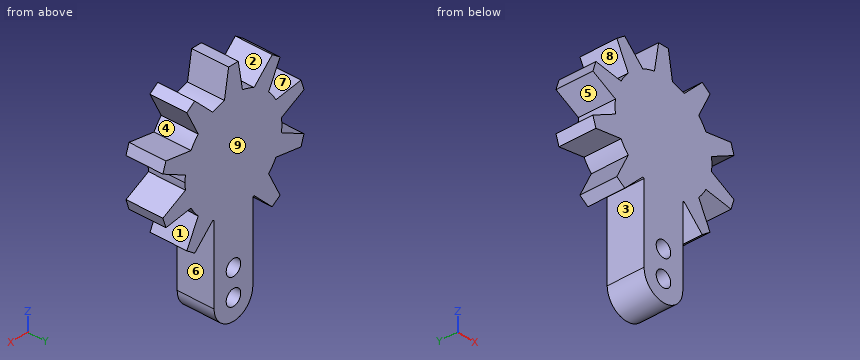
```python
from build123d import *

# Parameters (mm, degrees)
BOSS_EXTRUDE2_DEPTH = 7
SKETCH2_R           = 1.5
BOSS_EXTRUDE3_DEPTH = 7


with BuildPart() as part:
    # Sketch1 → Boss-Extrude2 (new body)
    with BuildSketch(Plane(origin=(0, 0, 0), x_dir=(1, 0, 0), z_dir=(0, 1, 0))):
        with BuildLine():
            Line((-2, 9), (-1.862495894, 9.825024633))
            ThreePointArc((-1.862495894, 9.825024633), (-3.090169944, 9.510565163), (-4.268213752, 9.043359518))
            Line((-4.268213752, 9.043359518), (-3.672033282, 8.456723454))
            Line((-3.672033282, 8.456723454), (-6.908101259, 6.105582445))
            Line((-6.908101259, 6.105582445), (-7.281795413, 6.853864279))
            ThreePointArc((-7.281795413, 6.853864279), (-8.090169944, 5.877852523), (-8.768610817, 4.807438439))
            Line((-8.768610817, 4.807438439), (-7.941474658, 4.683265982))
            Line((-7.941474658, 4.683265982), (-9.177542635, 0.879039917))
            Line((-9.177542635, 0.879039917), (-9.919696584, 1.264760725))
            ThreePointArc((-9.919696584, 1.264760725), (-10, 0), (-9.919696584, -1.264760725))
            Line((-9.919696584, -1.264760725), (-9.177542635, -0.879039917))
            Line((-9.177542635, -0.879039917), (-7.941474658, -4.683265982))
            Line((-7.941474658, -4.683265982), (-8.768610817, -4.807438439))
            ThreePointArc((-8.768610817, -4.807438439), (-8.090169944, -5.877852523), (-7.281795413, -6.853864279))
            Line((-7.281795413, -6.853864279), (-6.908101259, -6.105582445))
            Line((-6.908101259, -6.105582445), (-3.672033282, -8.456723454))
            Line((-3.672033282, -8.456723454), (-4.268213752, -9.043359518))
            ThreePointArc((-4.268213752, -9.043359518), (-3.090169944, -9.510565163), (-1.862495894, -9.825024633))
            Line((-1.862495894, -9.825024633), (-2, -9))
            Line((-2, -9), (2, -9))
            Line((2, -9), (1.862495894, -9.825024633))
            ThreePointArc((1.862495894, -9.825024633), (3.090169944, -9.510565163), (4.268213752, -9.043359518))
            Line((4.268213752, -9.043359518), (3.672033282, -8.456723454))
            Line((3.672033282, -8.456723454), (6.908101259, -6.105582445))
            Line((6.908101259, -6.105582445), (7.281795413, -6.853864279))
            ThreePointArc((7.281795413, -6.853864279), (8.090169944, -5.877852523), (8.768610817, -4.807438439))
            Line((8.768610817, -4.807438439), (7.941474658, -4.683265982))
            Line((7.941474658, -4.683265982), (9.177542635, -0.879039917))
            Line((9.177542635, -0.879039917), (9.919696584, -1.264760725))
            ThreePointArc((9.919696584, -1.264760725), (9.979903953, -0.633653756), (10, 0))
            ThreePointArc((10, 0), (9.979903953, 0.633653756), (9.919696584, 1.264760725))
            Line((9.919696584, 1.264760725), (9.177542635, 0.879039917))
            Line((9.177542635, 0.879039917), (7.941474658, 4.683265982))
            Line((7.941474658, 4.683265982), (8.768610817, 4.807438439))
            ThreePointArc((8.768610817, 4.807438439), (8.090169944, 5.877852523), (7.281795413, 6.853864279))
            Line((7.281795413, 6.853864279), (6.908101259, 6.105582445))
            Line((6.908101259, 6.105582445), (3.672033282, 8.456723454))
            Line((3.672033282, 8.456723454), (4.268213752, 9.043359518))
            ThreePointArc((4.268213752, 9.043359518), (3.090169944, 9.510565163), (1.862495894, 9.825024633))
            Line((1.862495894, 9.825024633), (2, 9))
            Line((2, 9), (-2, 9))
        make_face()
        with BuildLine():
            ThreePointArc((-8.768610817, -4.807438439), (-9.510565163, -3.090169944), (-9.919696584, -1.264760725))
            Line((-9.919696584, -1.264760725), (-14.574864739, -3.684198399))
            Line((-14.574864739, -3.684198399), (-13.95683075, -5.586311432))
            Line((-13.95683075, -5.586311432), (-8.768610817, -4.807438439))
        make_face()
        with BuildLine():
            ThreePointArc((-4.268213752, -9.043359518), (-5.877852523, -8.090169944), (-7.281795413, -6.853864279))
            Line((-7.281795413, -6.853864279), (-9.625795779, -11.547469663))
            Line((-9.625795779, -11.547469663), (-8.00776179, -12.723040168))
            Line((-8.00776179, -12.723040168), (-4.268213752, -9.043359518))
        make_face()
        with BuildLine():
            ThreePointArc((1.862495894, -9.825024633), (0, -10), (-1.862495894, -9.825024633))
            Line((-1.862495894, -9.825024633), (-1, -15))
            Line((-1, -15), (1, -15))
            Line((1, -15), (1.862495894, -9.825024633))
        make_face()
        with BuildLine():
            Line((9.625795779, -11.547469663), (7.281795413, -6.853864279))
            ThreePointArc((7.281795413, -6.853864279), (5.877852523, -8.090169944), (4.268213752, -9.043359518))
            Line((4.268213752, -9.043359518), (8.00776179, -12.723040168))
            Line((8.00776179, -12.723040168), (9.625795779, -11.547469663))
        make_face()
        with BuildLine():
            Line((14.574864739, -3.684198399), (9.919696584, -1.264760725))
            ThreePointArc((9.919696584, -1.264760725), (9.510565163, -3.090169944), (8.768610817, -4.807438439))
            Line((8.768610817, -4.807438439), (13.95683075, -5.586311432))
            Line((13.95683075, -5.586311432), (14.574864739, -3.684198399))
        make_face()
        with BuildLine():
            Line((13.95683075, 5.586311432), (8.768610817, 4.807438439))
            ThreePointArc((8.768610817, 4.807438439), (9.510565163, 3.090169944), (9.919696584, 1.264760725))
            Line((9.919696584, 1.264760725), (14.574864739, 3.684198399))
            Line((14.574864739, 3.684198399), (13.95683075, 5.586311432))
        make_face()
        with BuildLine():
            Line((8.00776179, 12.723040168), (4.268213752, 9.043359518))
            ThreePointArc((4.268213752, 9.043359518), (5.877852523, 8.090169944), (7.281795413, 6.853864279))
            Line((7.281795413, 6.853864279), (9.625795779, 11.547469663))
            Line((9.625795779, 11.547469663), (8.00776179, 12.723040168))
        make_face()
        with BuildLine():
            Line((1, 15), (-1, 15))
            Line((-1, 15), (-1.862495894, 9.825024633))
            ThreePointArc((-1.862495894, 9.825024633), (0, 10), (1.862495894, 9.825024633))
            Line((1.862495894, 9.825024633), (1, 15))
        make_face()
        with BuildLine():
            ThreePointArc((-7.281795413, 6.853864279), (-5.877852523, 8.090169944), (-4.268213752, 9.043359518))
            Line((-4.268213752, 9.043359518), (-8.00776179, 12.723040168))
            Line((-8.00776179, 12.723040168), (-9.625795779, 11.547469663))
            Line((-9.625795779, 11.547469663), (-7.281795413, 6.853864279))
        make_face()
        with BuildLine():
            ThreePointArc((-9.919696584, 1.264760725), (-9.510565163, 3.090169944), (-8.768610817, 4.807438439))
            Line((-8.768610817, 4.807438439), (-13.95683075, 5.586311432))
            Line((-13.95683075, 5.586311432), (-14.574864739, 3.684198399))
            Line((-14.574864739, 3.684198399), (-9.919696584, 1.264760725))
        make_face()
        with BuildLine():
            Line((-7.941474658, 4.683265982), (-8.768610817, 4.807438439))
            ThreePointArc((-8.768610817, 4.807438439), (-9.510565163, 3.090169944), (-9.919696584, 1.264760725))
            Line((-9.919696584, 1.264760725), (-9.177542635, 0.879039917))
            Line((-9.177542635, 0.879039917), (-7.941474658, 4.683265982))
        make_face()
        with BuildLine():
            Line((-2, -9), (-1.862495894, -9.825024633))
            ThreePointArc((-1.862495894, -9.825024633), (0, -10), (1.862495894, -9.825024633))
            Line((1.862495894, -9.825024633), (2, -9))
            Line((2, -9), (-2, -9))
        make_face()
        with BuildLine():
            ThreePointArc((4.268213752, -9.043359518), (5.877852523, -8.090169944), (7.281795413, -6.853864279))
            Line((7.281795413, -6.853864279), (6.908101259, -6.105582445))
            Line((6.908101259, -6.105582445), (3.672033282, -8.456723454))
            Line((3.672033282, -8.456723454), (4.268213752, -9.043359518))
        make_face()
        with BuildLine():
            Line((-6.908101259, -6.105582445), (-7.281795413, -6.853864279))
            ThreePointArc((-7.281795413, -6.853864279), (-5.877852523, -8.090169944), (-4.268213752, -9.043359518))
            Line((-4.268213752, -9.043359518), (-3.672033282, -8.456723454))
            Line((-3.672033282, -8.456723454), (-6.908101259, -6.105582445))
        make_face()
        with BuildLine():
            Line((-9.177542635, -0.879039917), (-9.919696584, -1.264760725))
            ThreePointArc((-9.919696584, -1.264760725), (-9.510565163, -3.090169944), (-8.768610817, -4.807438439))
            Line((-8.768610817, -4.807438439), (-7.941474658, -4.683265982))
            Line((-7.941474658, -4.683265982), (-9.177542635, -0.879039917))
        make_face()
        with BuildLine():
            Line((-3.672033282, 8.456723454), (-4.268213752, 9.043359518))
            ThreePointArc((-4.268213752, 9.043359518), (-5.877852523, 8.090169944), (-7.281795413, 6.853864279))
            Line((-7.281795413, 6.853864279), (-6.908101259, 6.105582445))
            Line((-6.908101259, 6.105582445), (-3.672033282, 8.456723454))
        make_face()
        with BuildLine():
            ThreePointArc((1.862495894, 9.825024633), (0, 10), (-1.862495894, 9.825024633))
            Line((-1.862495894, 9.825024633), (-2, 9))
            Line((-2, 9), (2, 9))
            Line((2, 9), (1.862495894, 9.825024633))
        make_face()
        with BuildLine():
            ThreePointArc((7.281795413, 6.853864279), (5.877852523, 8.090169944), (4.268213752, 9.043359518))
            Line((4.268213752, 9.043359518), (3.672033282, 8.456723454))
            Line((3.672033282, 8.456723454), (6.908101259, 6.105582445))
            Line((6.908101259, 6.105582445), (7.281795413, 6.853864279))
        make_face()
        with BuildLine():
            ThreePointArc((9.919696584, 1.264760725), (9.510565163, 3.090169944), (8.768610817, 4.807438439))
            Line((8.768610817, 4.807438439), (7.941474658, 4.683265982))
            Line((7.941474658, 4.683265982), (9.177542635, 0.879039917))
            Line((9.177542635, 0.879039917), (9.919696584, 1.264760725))
        make_face()
        with BuildLine():
            ThreePointArc((8.768610817, -4.807438439), (9.510565163, -3.090169944), (9.919696584, -1.264760725))
            Line((9.919696584, -1.264760725), (9.177542635, -0.879039917))
            Line((9.177542635, -0.879039917), (7.941474658, -4.683265982))
            Line((7.941474658, -4.683265982), (8.768610817, -4.807438439))
        make_face()
    extrude(amount=BOSS_EXTRUDE2_DEPTH)

    # Sketch2 → Boss-Extrude3 (add)
    with BuildSketch(Plane.XZ):
        with BuildLine():
            Line((-4, 0), (4, 0))
            Line((4, 0), (4, -24))
            ThreePointArc((4, -24), (0, -28), (-4, -24))
            Line((-4, -24), (-4, 0))
        make_face()
        with Locations(Location((0, -24, 0), (0, 0, 270))):
            Circle(SKETCH2_R, mode=Mode.SUBTRACT)
        with Locations(Location((0, -19, 0), (0, 0, 270))):
            Circle(SKETCH2_R, mode=Mode.SUBTRACT)
    extrude(amount=-BOSS_EXTRUDE3_DEPTH)


solid = part.part
```
Can you work these out from the model? Positions are in its coordinate system, mm. Face numbers are marked on the shaded views. A direction names the side the tool comes from. Round coordinates to 2 decimals unless told otherwise and drop trailing zeros. Loops run counter-clockwise (first coordinate to the right, second up) from the corner with the lowest first, then second, coordinate; pieces in that order, holes last. Notation, with made-up numbers: M 79.5,65.25 L 133.5,65.25 A24 ccw 133.5,79.25 Z; hole C 65.5,59 d3. An arc over 180 degrees is marked long. Answer as a JSON object with one key per item and string values. Group by question number.
Q1. Imagine slicing it at B-B, the plane z = -19. Please give me the cut outline in (x, y), then the cut area to 3 significant figures.
Q2. Imagine slicing it at D-D, the plane y = 5.75. Count the separate pieces of the cut face and the enclosed holes in it, then the cut area to 3 significant figures.
Q3. Imagine slicing it at A-A, the plane x = 0. Please give me the cut outline in (y, z), then the cut area to 3 significant figures.
Q4. Imagine slicing it at C-C, the plane x = 10.75. Please give me the cut outline in (y, z), then the cut area to 3 significant figures.
Q5. We'd pull the mould along X, two halves only. Please class the marked faces 6, 7, 8 and 9: +X half, -X half, draft (parallel to the pull), parting line (faces both ways), or undercut.
Q6. Will these pins go through, and if not, where does the flat tip stop? pin 1 (2 mm diameter, centred on y = 5.5, z = -21.5, fed in from -X); pin 2 (1.8 mm diameter, centred on x = 0, z = -24, fed in from -Y); pin 3 (1.5 mm diameter, centred on x = 11, y = 4, fed in from -Z) (3 decimals); pin 4 (1.5 mm diameter, centred on x = 9.5, y = 4, fed in from +Z).
Q7. Please list where these lines run through material, in increasing order: L1, parallel to X at y = 3.75, z = -19; L2, parallel to X at y = 6.5, z = 10.5; L3, parallel to Z at x = 8, y = 5.25.
Q8. On a 3-axis mill with a long thin cutter (end or side, diameter ignored), from which of +Z, -Z, +X, -X, +Y, -Y can I reach the whole of each face in a straight line? I mean the marked faces 1, 2, 3, 4 and 5. Say none if no direction works.
Findings:
{
 "1": {"outline": "M -4,0 L -1.5,0 L -1.5,7 L -4,7 Z; M 1.5,0 L 4,0 L 4,7 L 1.5,7 Z", "area": "35.0 mm2"},
 "2": {"separate pieces": "1", "enclosed holes": "2", "area": "569 mm2"},
 "3": {"outline": "M 0,-28 L 7,-28 L 7,-25.5 L 0,-25.5 Z; M 0,-22.5 L 7,-22.5 L 7,-20.5 L 0,-20.5 Z; M 0,-17.5 L 7,-17.5 L 7,15 L 0,15 Z", "area": "259 mm2"},
 "4": {"outline": "M 0,-5.1 L 7,-5.1 L 7,-1.7 L 0,-1.7 Z; M 0,1.7 L 7,1.7 L 7,5.1 L 0,5.1 Z", "area": "47.7 mm2"},
 "5": {"face 6": "undercut", "face 7": "undercut", "face 8": "-X half", "face 9": "draft"},
 "6": {"pin 1": "stops at x = -4", "pin 2": "passes through", "pin 3": "stops at z = -5.255", "pin 4": "stops at z = 12.18"},
 "7": {"L1": "x = -4 to -1.5, 1.5 to 4", "L2": "x = -9.1 to -5.75, -1.75 to 1.75, 5.75 to 9.1", "L3": "z = -12.72 to -8.29, -6 to 6, 8.29 to 12.72"},
 "8": {"face 1": "+X, +Y, -Y", "face 2": "+Z, +Y, -Y", "face 3": "-Z, +Y, -Y", "face 4": "+Y, -Y", "face 5": "-X, +Y, -Y"}
}
